```python
from build123d import *

# Parameters (mm, degrees)
F0_W     = 25.4
F0_H     = 50.8
F1_DEPTH = 12.7
F2_W     = 25.4
F2_H     = 19.9644
F3_DEPTH = 3.175
F5_D     = 4.0386


with BuildPart() as f1:
    # F0 (on Top) → F1 (new body)
    with BuildSketch(Plane.XY):
        Rectangle(F0_W, F0_H)
    extrude(amount=F1_DEPTH)

    # F2 (on face) → F3 (cut)
    with BuildSketch(Plane.XY.offset(12.7)):
        Rectangle(F2_W, F2_H)
    extrude(amount=-F3_DEPTH, mode=Mode.SUBTRACT)

    # F5 (through all)
    with Locations(Plane.XY.offset(12.7)):
        with Locations((0, 13.7922), (0, -13.7922)):
            Hole(F5_D / 2)


solid = f1.part
```
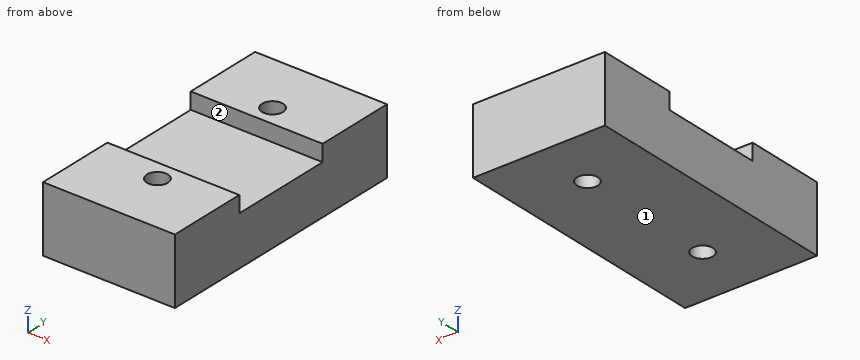
Geometry check sheet. Reference: the model listing, model coordinates, mm. Face numbers are marked on the shaded views. A direction names the side the tool comes from. Round coordinates to 2 decimals unless told otherwise and drop trailing zeros. Order: outer loops, then holes, each group sorted by start corner. A loop starts at its lowest first (then second) coordinate and runs counter-clockwise, first axis right, second up. Notation, with made-up numbers: (-21.75, 12) - (-12.75, 12) arc R25 cw to (-12.75, 29) - close; hole circle Ø5 at (11, 71.5). An arc over 180 degrees is marked (long way). Use a Markdown table: item, result. Add a question column.
1) Thickness scan on line 1 along Y through (x, z) = (0, 4.5); line 2 along Y through (x, z) = (1.5, 3); line 3 along Z through (x, y) = (-4.75, 8.5) (3 decimals). Record the ranges inside material, lowest first.
2) Section check A-A (x = 0). Record the cut outline in (y, z) (1 decimal).
3) Section check C-C (x = 9.75). Record the cut outline in (y, z) (3 decimals).
4) Section check B-B (z = 10). Record the cut outline in (x, y).
5) Gauge pin test, flat ends, axial feed: P1, Ø2.5, axis at x = 0, y = 13.79, coming from the +Z side; P2, Ø10, axis at x = -1, y = -2.5, coming from the +Z side (3 decimals). Record the tip position at first contact, or that the pin passes through.
6) Section check D-D (y = 3). Record the cut outline in (x, z) (3 decimals).
7) Set-up check for the marked faces 1 and 2: record each of +Z, -Z, +X, -X, +Y, -Y from which the full face is reachable in a straight line by a thin tool's end or side.
Established:
| question | item | result |
|---|---|---|
| 1 | line 1 | -25.4 to -15.81, -11.77 to 11.77, 15.81 to 25.4 |
| 1 | line 2 | -25.4 to -15.14, -12.44 to 12.44, 15.14 to 25.4 |
| 1 | line 3 | 0 to 9.525 |
| 2 | outline | (-25.4, 0) - (-15.8, 0) - (-15.8, 12.7) - (-25.4, 12.7) - close; (-11.8, 0) - (11.8, 0) - (11.8, 12.7) - (10, 12.7) - (10, 9.5) - (-10, 9.5) - (-10, 12.7) - (-11.8, 12.7) - close; (15.8, 0) - (25.4, 0) - (25.4, 12.7) - (15.8, 12.7) - close |
| 3 | outline | (-25.4, 0) - (25.4, 0) - (25.4, 12.7) - (9.982, 12.7) - (9.982, 9.525) - (-9.982, 9.525) - (-9.982, 12.7) - (-25.4, 12.7) - close |
| 4 | outline | (-12.7, -25.4) - (12.7, -25.4) - (12.7, -9.98) - (-12.7, -9.98) - close; (-12.7, 9.98) - (12.7, 9.98) - (12.7, 25.4) - (-12.7, 25.4) - close; hole circle Ø4.04 at (0, -13.79); hole circle Ø4.04 at (0, 13.79) |
| 5 | P1 | through |
| 5 | P2 | z = 9.525 |
| 6 | outline | (-12.7, 0) - (12.7, 0) - (12.7, 9.525) - (-12.7, 9.525) - close |
| 7 | face 1 | -Z, +X, -X, +Y, -Y |
| 7 | face 2 | +Z, +X, -X |
